from build123d import *

# Parameters (mm, degrees)
F0_R     = 45.5
F0_R_2   = 2.75
F0_R_3   = 2.05
F0_R_4   = 22
F1_DEPTH = 12
F3_DEPTH = 5.1


# Not quite as in the source:
# - a feature names something its author has since deleted; it is built from what else it names


with BuildPart() as f1:
    # F0 (on Top) → F1 (new body)
    with BuildSketch(Plane.XY):
        Circle(F0_R)
        with Locations((-18, -31.1769145362)):
            Circle(F0_R_2, mode=Mode.SUBTRACT)
        with Locations((-24.7683265482, -14.3)):
            Circle(F0_R_3, mode=Mode.SUBTRACT)
        with Locations((0, -28.6)):
            Circle(F0_R_3, mode=Mode.SUBTRACT)
        with Locations((18, -31.1769145362)):
            Circle(F0_R_2, mode=Mode.SUBTRACT)
        with Locations((24.7683265482, -14.3)):
            Circle(F0_R_3, mode=Mode.SUBTRACT)
        with Locations((-36, 0)):
            Circle(F0_R_2, mode=Mode.SUBTRACT)
        with Locations((-24.7683265482, 14.3)):
            Circle(F0_R_3, mode=Mode.SUBTRACT)
        with Locations((-18, 31.1769145362)):
            Circle(F0_R_2, mode=Mode.SUBTRACT)
        Circle(F0_R_4, mode=Mode.SUBTRACT)
        with Locations((36, 0)):
            Circle(F0_R_2, mode=Mode.SUBTRACT)
        with Locations((24.7683265482, 14.3)):
            Circle(F0_R_3, mode=Mode.SUBTRACT)
        with Locations((0, 28.6)):
            Circle(F0_R_3, mode=Mode.SUBTRACT)
        with Locations((18, 31.1769145362)):
            Circle(F0_R_2, mode=Mode.SUBTRACT)
    extrude(amount=F1_DEPTH)

    # F2 (on face) → F3 (cut)
    with BuildSketch(Plane.XY.offset(12)):
        with BuildLine():
            ThreePointArc((-20.4683265482, 14.3), (-20.9661824008, 16.3084072998), (-22.3444660282, 17.8517460747))
            ThreePointArc((-22.3444660282, 17.8517460747), (-23.0302843715, 16.957771132), (-23.6803579094, 16.0374764001))
            ThreePointArc((-23.6803579094, 16.0374764001), (-22.9748891072, 15.2930166893), (-22.7183265482, 14.3))
            ThreePointArc((-22.7183265482, 14.3), (-23.7116725089, 12.5433036002), (-25.7290409298, 12.4890533202))
            ThreePointArc((-25.7290409298, 12.4890533202), (-26.2010027777, 11.4659257561), (-26.6322986167, 10.425002177))
            ThreePointArc((-26.6322986167, 10.425002177), (-22.4797767776, 10.6595961835), (-20.4683265482, 14.3))
        make_face()
        with BuildLine():
            ThreePointArc((-23.6803579094, 16.0374764001), (-23.0302843715, 16.957771132), (-22.3444660282, 17.8517460747))
            ThreePointArc((-22.3444660282, 17.8517460747), (-28.4922357845, 16.45), (-26.6322986167, 10.425002177))
            ThreePointArc((-26.6322986167, 10.425002177), (-26.2010027777, 11.4659257561), (-25.7290409298, 12.4890533202))
            ThreePointArc((-25.7290409298, 12.4890533202), (-26.543678626, 15.325), (-23.6803579094, 16.0374764001))
        make_face()
        with BuildLine():
            ThreePointArc((2.0486830204, 28.5265297203), (3.1707184061, 28.4236968881), (4.2878325885, 28.2767482517))
            ThreePointArc((4.2878325885, 28.2767482517), (4.2969570705, 28.438259669), (4.3, 28.6))
            ThreePointArc((4.3, 28.6), (-0.161740331, 32.8969570705), (-4.2878325885, 28.2767482517))
            ThreePointArc((-4.2878325885, 28.2767482517), (-3.1707184061, 28.4236968881), (-2.0486830204, 28.5265297203))
            ThreePointArc((-2.0486830204, 28.5265297203), (-0.0367410412, 30.6496707287), (2.05, 28.6))
            ThreePointArc((2.05, 28.6), (2.0496707287, 28.5632589588), (2.0486830204, 28.5265297203))
        make_face()
        with BuildLine():
            ThreePointArc((-4.2878325885, 28.2767482517), (0, 24.3), (4.2878325885, 28.2767482517))
            ThreePointArc((4.2878325885, 28.2767482517), (3.1707184061, 28.4236968881), (2.0486830204, 28.5265297203))
            ThreePointArc((2.0486830204, 28.5265297203), (0, 26.55), (-2.0486830204, 28.5265297203))
            ThreePointArc((-2.0486830204, 28.5265297203), (-3.1707184061, 28.4236968881), (-4.2878325885, 28.2767482517))
        make_face()
        with BuildLine():
            ThreePointArc((25.7290409298, 12.4890533202), (26.2010027777, 11.4659257561), (26.6322986167, 10.425002177))
            ThreePointArc((26.6322986167, 10.425002177), (28.4087303647, 12.0114502293), (29.0683265482, 14.3))
            ThreePointArc((29.0683265482, 14.3), (26.776733848, 18.1021441475), (22.3444660282, 17.8517460747))
            ThreePointArc((22.3444660282, 17.8517460747), (23.0302843715, 16.957771132), (23.6803579094, 16.0374764001))
            ThreePointArc((23.6803579094, 16.0374764001), (25.7613432375, 16.093437441), (26.8183265482, 14.3))
            ThreePointArc((26.8183265482, 14.3), (26.525022948, 13.2433459606), (25.7290409298, 12.4890533202))
        make_face()
        with BuildLine():
            ThreePointArc((22.3444660282, 17.8517460747), (21.044417312, 12.15), (26.6322986167, 10.425002177))
            ThreePointArc((26.6322986167, 10.425002177), (26.2010027777, 11.4659257561), (25.7290409298, 12.4890533202))
            ThreePointArc((25.7290409298, 12.4890533202), (22.9929744705, 13.275), (23.6803579094, 16.0374764001))
            ThreePointArc((23.6803579094, 16.0374764001), (23.0302843715, 16.957771132), (22.3444660282, 17.8517460747))
        make_face()
        with BuildLine():
            ThreePointArc((29.0683265482, -14.3), (28.4087303647, -12.0114502293), (26.6322986167, -10.425002177))
            ThreePointArc((26.6322986167, -10.425002177), (26.2010027777, -11.4659257561), (25.7290409298, -12.4890533202))
            ThreePointArc((25.7290409298, -12.4890533202), (26.525022948, -13.2433459606), (26.8183265482, -14.3))
            ThreePointArc((26.8183265482, -14.3), (25.7613432375, -16.093437441), (23.6803579094, -16.0374764001))
            ThreePointArc((23.6803579094, -16.0374764001), (23.0302843715, -16.957771132), (22.3444660282, -17.8517460747))
            ThreePointArc((22.3444660282, -17.8517460747), (26.776733848, -18.1021441475), (29.0683265482, -14.3))
        make_face()
        with BuildLine():
            ThreePointArc((25.7290409298, -12.4890533202), (26.2010027777, -11.4659257561), (26.6322986167, -10.425002177))
            ThreePointArc((26.6322986167, -10.425002177), (21.044417312, -12.15), (22.3444660282, -17.8517460747))
            ThreePointArc((22.3444660282, -17.8517460747), (23.0302843715, -16.957771132), (23.6803579094, -16.0374764001))
            ThreePointArc((23.6803579094, -16.0374764001), (22.9929744705, -13.275), (25.7290409298, -12.4890533202))
        make_face()
        with BuildLine():
            ThreePointArc((2.0486830204, -28.5265297203), (3.1707184061, -28.4236968881), (4.2878325885, -28.2767482517))
            ThreePointArc((4.2878325885, -28.2767482517), (0, -24.3), (-4.2878325885, -28.2767482517))
            ThreePointArc((-4.2878325885, -28.2767482517), (-3.1707184061, -28.4236968881), (-2.0486830204, -28.5265297203))
            ThreePointArc((-2.0486830204, -28.5265297203), (0, -26.55), (2.0486830204, -28.5265297203))
        make_face()
        with BuildLine():
            ThreePointArc((4.3, -28.6), (4.2969570705, -28.438259669), (4.2878325885, -28.2767482517))
            ThreePointArc((4.2878325885, -28.2767482517), (3.1707184061, -28.4236968881), (2.0486830204, -28.5265297203))
            ThreePointArc((2.0486830204, -28.5265297203), (2.0496707287, -28.5632589588), (2.05, -28.6))
            ThreePointArc((2.05, -28.6), (-0.0367410412, -30.6496707287), (-2.0486830204, -28.5265297203))
            ThreePointArc((-2.0486830204, -28.5265297203), (-3.1707184061, -28.4236968881), (-4.2878325885, -28.2767482517))
            ThreePointArc((-4.2878325885, -28.2767482517), (-0.161740331, -32.8969570705), (4.3, -28.6))
        make_face()
        with BuildLine():
            ThreePointArc((-23.6803579094, -16.0374764001), (-23.0302843715, -16.957771132), (-22.3444660282, -17.8517460747))
            ThreePointArc((-22.3444660282, -17.8517460747), (-20.9661824008, -16.3084072998), (-20.4683265482, -14.3))
            ThreePointArc((-20.4683265482, -14.3), (-22.4797767776, -10.6595961835), (-26.6322986167, -10.425002177))
            ThreePointArc((-26.6322986167, -10.425002177), (-26.2010027777, -11.4659257561), (-25.7290409298, -12.4890533202))
            ThreePointArc((-25.7290409298, -12.4890533202), (-23.7116725089, -12.5433036002), (-22.7183265482, -14.3))
            ThreePointArc((-22.7183265482, -14.3), (-22.9748891072, -15.2930166893), (-23.6803579094, -16.0374764001))
        make_face()
        with BuildLine():
            ThreePointArc((-26.6322986167, -10.425002177), (-28.4922357845, -16.45), (-22.3444660282, -17.8517460747))
            ThreePointArc((-22.3444660282, -17.8517460747), (-23.0302843715, -16.957771132), (-23.6803579094, -16.0374764001))
            ThreePointArc((-23.6803579094, -16.0374764001), (-26.543678626, -15.325), (-25.7290409298, -12.4890533202))
            ThreePointArc((-25.7290409298, -12.4890533202), (-26.2010027777, -11.4659257561), (-26.6322986167, -10.425002177))
        make_face()
    extrude(amount=-F3_DEPTH, mode=Mode.SUBTRACT)


solid = f1.part
Verification items for the finished model (mm, model axes). A direction names the side the tool comes from. Give positions to 0.01 mm unless a question says otherwise; leave off trailing zeros. Loops run counter-clockwise (first coordinate to the right, second up) from the corner with the lowest first, then second, coordinate; pieces in that order, holes last.
1) Draft check along X on faces 1 (the cylindrical face through (17.64, -28.45, 5.92)), 2 (the flat face through (-11, -20, 0)), 3 (the cylindrical face through (-36.107, -27.686, 5.916)). Enter one of: pulls with the +X half, pulls with the -X half, needs draft (parallel to the pull), parting line crosses it, or undercut.
2) Depth check by flat-ended pin: pin 1 Ø4 at (y, z) = (-5.5, 4.5) entering from +X; pin 2 Ø6.5 at (x, y) = (-24.77, 14.3) entering from +Z; pin 3 Ø9.5 at (x, y) = (24, -14) entering from +Z; pin 4 Ø4 at (x, z) = (-29.5, 8) entering from +Y. Enter the tip coordinate at first touch or a pass-through.
3) Set-up check for faces 4 (the cylindrical face through (-18.36, -28.45, 5.92)), 5 (the flat face through (-24, 12, 6.9)): record each of +Z, -Z, +X, -X, +Y, -Y from which the full face is reachable in a straight line by a thin tool's end or side.
4) Sectioned sample at A-A, the plane x = -36. Enter the section's corners in (y, z).
5) Sectioned sample at D-D, the plane z = 2. Count the separate pieces of the cut face and the enclosed holes in it, then the cut area to 3 significant figures.
6) Sectioned sample at C-C, the plane x = -18. Enter the section's corners in (y, z).
7) Thickness scan on line 1 along X through (y, z) = (14.3, 2.75); line 2 along Y through (x, z) = (-25.5, 8); line 3 along Y through (x, z) = (18, 3). Record the ranges inside material, lowest first.
8) Sectioned sample at B-B, the plane y = 0. Enter the section's corners in (x, z), then the cut area to 3 significant figures.
Answers:
1. face 1: undercut
1. face 2: needs draft
1. face 3: parting line crosses it
2. pin 1: stops at x = 45.37
2. pin 2: stops at z = 6.9
2. pin 3: stops at z = 12
2. pin 4: stops at y = 36.25
3. face 4: +Z, -Z
3. face 5: +Z
4. outline: (-27.83, 0) - (-2.75, 0) - (-2.75, 12) - (-27.83, 12) - close; (2.75, 0) - (27.83, 0) - (27.83, 12) - (2.75, 12) - close
5. separate pieces: 1
5. enclosed holes: 13
5. area: 4,760 mm2
6. outline: (-41.79, 0) - (-33.93, 0) - (-33.93, 12) - (-41.79, 12) - close; (-28.43, 0) - (-12.65, 0) - (-12.65, 12) - (-28.43, 12) - close; (12.65, 0) - (28.43, 0) - (28.43, 12) - (12.65, 12) - close; (33.93, 0) - (41.79, 0) - (41.79, 12) - (33.93, 12) - close
7. line 1: x = -43.19 to -26.82, -22.72 to -16.72, 16.72 to 22.72, 26.82 to 43.19
7. line 2: y = -37.68 to -18.54, -10.06 to 10.06, 18.54 to 37.68
7. line 3: y = -41.79 to -33.93, -28.43 to -12.65, 12.65 to 28.43, 33.93 to 41.79
8. outline: (-45.5, 0) - (-38.75, 0) - (-38.75, 12) - (-45.5, 12) - close; (-33.25, 0) - (-22, 0) - (-22, 12) - (-33.25, 12) - close; (22, 0) - (33.25, 0) - (33.25, 12) - (22, 12) - close; (38.75, 0) - (45.5, 0) - (45.5, 12) - (38.75, 12) - close
8. area: 432 mm2
